Autodesk Inventor part; units mm, degrees
ref_plane "YZ Plane" through (0, 0, 0) normal (1, 0, 0) x (0, 1, 0)
ref_plane "XZ Plane" through (0, 0, 0) normal (0, 1, 0) x (-1, 0, 0)
ref_plane "XY Plane" through (0, 0, 0) normal (0, 0, 1) x (1, 0, 0)
sketch "Sketch1" plane through (0, 0, 0) normal (0, 1, 0) x (-1, 0, 0)
  line L0 (0, 0) -> (62.3538, -36)
  line L1 (0, 25) -> (0, -25) construction
  line L2 (62.3538, -36) -> (59.6038, -40.7631)
  line L3 (59.6038, -40.7631) -> (16.2879, -15.7547)
  line L4 (16.2879, -15.7547) -> (0, -43.9661)
  line L5 (0, 0) -> (0, -43.9661)
  dimension "d0" = 72
  dimension "d1" = 50
  dimension "d2" = 60
  dimension "d3" = 5.5
  dimension "d19" = 90
extrude "Extrusion1" add sketch "Sketch1" along normal blind 72
sketch "Sketch2" plane through (0, 0, 0) normal (-0.5, 0, 0.866) x (0.866, 0, 0.5)
  line L0 (-62, 10.875) -> (-36.83, 10.875)
  line L1 (-36.83, 10.875) -> (-36.83, 61.125)
  line L2 (-36.83, 61.125) -> (-62, 61.125)
  line L3 (-62, 61.125) -> (-62, 10.875)
  line L4 (-72, 0) -> (-72, 72)
  circle A0 centre (-61.8, 2.155) radius 1
  point P0 (0, 0)
  point P1 (-62, 36)
  point P2 (-72, 36)
  dimension "d6" = 25.17
  dimension "d7" = 50.25
  dimension "d8" = 10
  dimension "d66" = 2
  dimension "d67" = 8.72
  dimension "d68" = 0.2
extrude "Extrusion2" cut sketch "Sketch2" against normal up to surface (5.5 mm away)
sketch "Sketch3" plane through (-59.6038, 0, -40.7631) normal (0.5, 0, -0.866) x (-0.866, 0, -0.5)
  line L0 (-6.585, 63.785) -> (-38.585, 63.785)
  line L1 (-38.585, 63.785) -> (-38.585, -1.215)
  line L2 (-38.585, -1.215) -> (-6.585, -1.215)
  line L3 (-6.585, -1.215) -> (-6.585, 63.785)
  line L4 (-35.17, 61.125) -> (-10, 61.125)
  point P0 (-72, 0)
  point P1 (-22.585, 63.785)
  point P2 (-22.585, 61.125)
  dimension "d11" = 32
  dimension "d12" = 65
  dimension "d13" = 2.66
extrude "Extrusion3" cut sketch "Sketch3" against normal blind 4.5
fillet "Fillet1" radius 3 1 edges at (0, 36, 0)
fillet "Fillet2" radius 2 1 edges at (0, 36, -43.9661)
fillet "Fillet3" radius 4 2 edges at (-60.9788, 72, -38.3816) (-60.9788, 0, -38.3816)
fillet "Fillet4" radius 4 1 edges at (-16.2879, 36, -15.7547)
sketch "Sketch4" plane through (-26.1882, 0, -21.4706) normal (0.5, 0, -0.866) x (-0.866, 0, -0.5)
  circle A0 centre (35.085, 16.41) radius 1.55
  line L0 (38.585, 4) -> (38.585, 68)
  circle A1 centre (35.085, 47.41) radius 1.55
  circle A2 centre (-2.915, 16.41) radius 1.6
  circle A3 centre (-2.915, 47.41) radius 1.6
  point P0 (-33.415, 0)
  point P1 (34.585, 0)
  dimension "d21" = 3.1
  dimension "d22" = 16.41
  dimension "d23" = 3.5
  dimension "d24" = 3.1
  dimension "d25" = 31
  dimension "d26" = 3.2
  dimension "d27" = 38
  dimension "d28" = 3.2
  dimension "d29" = 38
extrude "Extrusion4" cut sketch "Sketch4" against normal up to surface (4.5 mm away)
sketch "Sketch5" plane through (0, 0, 0) normal (0, -1, 0) x (1, 0, 0)
  line L0 (-11.1256, -19.2586) -> (-11.1256, -9.2074) construction
  line L1 (-11.1256, -9.2074) -> (-1.0319, -9.2074) construction
  line L2 (-1.0319, -9.2074) -> (-1.0319, -19.2586) construction
  line L3 (-1.0319, -19.2586) -> (-11.1256, -19.2586) construction
  arc A0 (-8.7423, -17.7336) -> (-8.7372, -10.7469) centre (-6.0502, -14.2422) ccw
  arc A1 (-9.1232, -18.214) -> (-9.1477, -10.2896) centre (-6.0502, -14.2422) ccw
  arc A2 (-9.1477, -10.2896) -> (-8.7372, -10.7469) centre (-8.8163, -10.405) ccw
  arc A3 (-8.7423, -17.7336) -> (-9.1232, -18.214) centre (-8.8713, -18.0225) ccw
  line L4 (-4.6557, -14.5422) -> (-7.2177, -14.5422)
  line L5 (-7.2177, -14.5422) -> (-7.2177, -13.9533)
  line L6 (-7.2177, -13.9533) -> (-4.6557, -13.9533)
  line L7 (-4.6557, -13.9533) -> (-4.6557, -14.5422)
  arc A4 (-4.6557, -14.5422) -> (-4.6557, -13.9533) centre (-4.7199, -14.2478) ccw
  arc A5 (-7.2177, -13.9533) -> (-7.2177, -14.5422) centre (-7.171, -14.2478) ccw
  arc A6 (-8.2247, -12.6322) -> (-8.1705, -15.9511) centre (-6.0663, -14.2568) ccw
  arc A7 (-7.7175, -12.932) -> (-7.6745, -15.6001) centre (-6.057, -14.2396) ccw
  arc A8 (-8.6126, -12.2607) -> (-8.5782, -16.3059) centre (-6.0095, -14.2613) ccw
  arc A9 (-9.1192, -11.9337) -> (-9.0775, -16.6329) centre (-6.1136, -14.2568) ccw
  arc A10 (-9.5852, -11.4861) -> (-9.568, -17.0116) centre (-5.9362, -14.2375) ccw
  point P0 (0, 0)
properties part number "ShelfLabelStand"
Can you work these out from the model? Positions are in its coordinate system, mm. A direction names the side the tool comes from. Give positions to 0.01 mm unless a question says otherwise; leave off trailing zeros. Loops run counter-clockwise (first coordinate to the right, second up) from the corner with the lowest first, then second, coordinate; pieces in that order, holes last. Notation, with made-up numbers: M 42,58 L 62,58 A20 cw 62,78 Z; hole C 54,57 d3. An arc over 180 degrees is marked long. One line per item, written item: value.
1) On a 3-axis mill with a long thin cutter (end or side, diameter ignored), from which of +Z, -Z, +X, -X, +Y, -Y can I reach the whole of each face in a straight line? I mean faces 5 (the face through (-55.01, 31.45, -35.55)), 6 (the face through (-9.084, 35.496, -28.232)), 7 (the face through (-12, 0, -20)), 8 (the face through (-25.895, 47.432, -16.103)). Say none if no direction works.
Geometry check:
face 5: -Y
face 6: -Z, +Y, -Y
face 7: +Z, -Z, +X, -X, -Y
face 8: none
2) Thinking about a two-plate mould opening in Z: for faces 1 (the face through (-57.391, 14.897, -36.923)), 2 (the face through (-26.59, 35.5, -15.35)), 3 (the face through (-25.01, 43.83, -20.79)), 4 (the face through (-42, 61.125, -25)), which applies, +Z half, -Z half, draft (parallel to the pull), parting line (faces both ways), or undercut?
Geometry check:
face 1: undercut
face 2: +Z half
face 3: -Z half
face 4: draft
3) Imagine slicing it at C-C on y = 6. Write out the boundary of the cut face in (x, z), and give its area (3 significant figures).
Geometry check:
outline: M -62.35,-36 L -59.6,-40.76 L -53.9,-37.47 L -56.15,-33.57 L -28.44,-17.57 L -26.19,-21.47 L -19.75,-17.75 A4 cw -14.29,-19.22 L -3.73,-37.5 A2 ccw 0,-36.5 L 0,-5.2 A3 ccw -4.5,-2.6 Z
area: 537 mm²
4) Please list where these lines run through material, in increasing order: line 1 (X direction, y = 47, z = -18); line 2 (X direction, y = 41, z = -37.5); line 3 (Y direction, x = -50, z = -35) (3 decimals).
Geometry check:
line 1: x = -31.18 to -29.18, -28.19 to -26.61, -23.04 to -20.18, -15.38 to 0
line 2: x = -61.49 to -53.95, -3.73 to -0.27
line 3: y = 63.785 to 72
5) Imagine slicing it at B-B on x = -50. Write out the boundary of the cut face in (y, z) (3 decimals), and give its area (3 significant figures).
Geometry check:
outline: M 0,-30.02 L 10.875,-30.02 L 10.875,-28.868 L 0,-28.868 Z; M 61.125,-30.02 L 63.785,-30.02 L 63.785,-35.218 L 72,-35.218 L 72,-28.868 L 61.125,-28.868 Z
area: 67.8 mm²
6) I'm going to push flat-ended pins straight in: pin 1 (10 mm diameter, centred on y = 10.5, z = -26.5, fed in from +X); pin 2 (8 mm diameter, centred on y = 35.5, z = -35, fed in from -X); pin 3 (1 mm diameter, centred on x = -18.5, y = 53, fed in from -Z). Where does each tip first touch, or does it pass through?
Geometry check:
pin 1: stops at x = 0
pin 2: stops at x = -62.35
pin 3: stops at z = -17.42
7) Imagine slicing it at D-D on x = -29.5. Write out the boundary of the cut face in (y, z) (3 decimals), and give its area (3 significant figures).
Geometry check:
outline: M 0,-18.184 L 63.785,-18.184 L 63.785,-23.383 L 72,-23.383 L 72,-17.032 L 0,-17.032 Z
area: 126 mm²
8) Imagine slicing it at A-A on y = 55.5. Write out the boundary of the cut face in (x, z) (3 decimals), and give its area (3 significant figures).
Geometry check:
outline: M -62.354,-36 L -59.604,-40.763 L -53.901,-37.471 L -56.152,-33.572 L -53.195,-31.864 L -53.694,-31 Z; M -31.896,-18.415 L -31.397,-19.279 L -28.439,-17.572 L -26.188,-21.471 L -19.752,-17.755 A4 cw -14.288,-19.219 L -3.732,-37.502 A2 ccw 0,-36.502 L 0,-5.196 A3 ccw -4.5,-2.598 Z
area: 512 mm²
